Source: CAD feature listing. Evaluate the final solid. Frame: model axes, mm. A direction names the side the tool comes from. Round coordinates to 2 decimals unless told otherwise and drop trailing zeros. Write each loop counter-clockwise with the first axis right and the second up, starting at its lowest first coordinate (ties: lowest second). Pieces come first, ordered by that corner, then holes.
from build123d import *

# Parameters (mm, degrees)
SKETCH_1_R      = 1.65
EXTRUDE_1_DEPTH = 5
FILLET_2_R      = 4
FILLET_3_R      = 40
FILLET_4_R      = 10
EXTRUDE_2_DEPTH = 55


with BuildPart() as part:
    # 草图1 → 凸台-拉伸1 (new body)
    with BuildSketch(Plane.XY):
        with BuildLine():
            Line((-11.5, 79.5), (-11.5, 82))
            ThreePointArc((-11.5, 82), (6.103622298, 73.512939805), (10.426977744, 54.454442843))
            Line((10.426977744, 54.454442843), (13.41461423, 33.96926032))
            Line((13.41461423, 33.96926032), (11.539893904, 12.741041785))
            Line((11.539893904, 12.741041785), (4.278741136, 12.025251419))
            Line((4.278741136, 12.025251419), (-1.047111461, 14.664575003))
            Line((-1.047111461, 14.664575003), (3.709660575, 42.919402146))
            ThreePointArc((3.709660575, 42.919402146), (1.596827744, 41.204560595), (-0.707567867, 39.757320125))
            Line((-0.707567867, 39.757320125), (-1.906726993, 41.950951222))
            ThreePointArc((-1.906726993, 41.950951222), (7.877576933, 64.450708254), (-11.5, 79.5))
        make_face()
        with Locations((5.679475492, 16.683750627)):
            Circle(SKETCH_1_R, mode=Mode.SUBTRACT)
        with Locations((8.382327473, 29.399669437)):
            Circle(SKETCH_1_R, mode=Mode.SUBTRACT)
    extrude(amount=EXTRUDE_1_DEPTH)

    # 圆角2
    fillet_2_edges = [part.edges().sort_by_distance(p)[0] for p in [
        (10.426977744, 54.454442843, 2.5),
    ]]
    fillet(fillet_2_edges, radius=FILLET_2_R)

    # 圆角3
    fillet_3_edges = [part.edges().sort_by_distance(p)[0] for p in [
        (13.41461423, 33.96926032, 2.5),
    ]]
    fillet(fillet_3_edges, radius=FILLET_3_R)

    # 圆角4
    fillet_4_edges = [part.edges().sort_by_distance(p)[0] for p in [
        (4.278741136, 12.025251419, 2.5),
    ]]
    fillet(fillet_4_edges, radius=FILLET_4_R)

    # 草图2 → 凸台-拉伸2 (add)
    with BuildSketch(Plane(origin=(0, 0, 0), x_dir=(-1, 0, 0), z_dir=(0, 0, -1))):
        with BuildLine():
            Line((11.5, 82), (11.5, 79.5))
            ThreePointArc((11.5, 79.5), (-7.877576933, 64.450708254), (1.906726993, 41.950951222))
            Line((1.906726993, 41.950951222), (0.707567867, 39.757320125))
            ThreePointArc((0.707567867, 39.757320125), (-10.299774049, 65.069546786), (11.5, 82))
        make_face()
    extrude(amount=-EXTRUDE_2_DEPTH)


solid = part.part
1) Section query D-D on y = 74.5. Return the cut outline in (x, z).
Taken from the geometry:
outline: (1.73, 0) - (5.27, 0) - (5.27, 55) - (1.73, 55) - close
2) Section query C-C on y = 48.5. Return the cut outline in (x, z).
Taken from the geometry:
outline: (5.2, 0) - (11.3, 0) - (11.3, 5) - (8.13, 5) - (8.13, 55) - (5.2, 55) - close
3) Contact query for flat-ended pins moving along their axis: P1, Ø3, axis at y = 50, z = 7, coming from the -X side; P2, Ø1, axis at x = 4, y = 19.5, coming from the +Z side; P3, Ø1, axis at x = 4.5, z = 21.5, coming from the -Y side. Output: stop coordinate, or through.
Taken from the geometry:
P1: stops at x = 5.2
P2: stops at z = 5
P3: stops at y = 43.19
4) Pull-direction query (Y, two-part tool) for faces 1 (the face through (8.02, 27.79, 2.46)), 2 (the face through (9.367, 12.527, 2.465)), 3 (the face through (5, 37, 0)); classes: released by +Y, released by -Y, zero draft, split by the parting line, or undercut.
Taken from the geometry:
face 1: undercut
face 2: released by -Y
face 3: zero draft
5) Section query B-B on z = 42. Return the cut outline in (x, y).
Taken from the geometry:
outline: (-11.5, 79.5) arc R20 cw to (-1.91, 41.95) - (-0.71, 39.76) arc R22.5 ccw to (-11.5, 82) - close
6) Reachability of faces 4 (the face through (11.62, 46.28, 2.46)), 5 (the face through (-11.5, 81, 27)), 6 (the face through (6, 29, 5)) from +Z, -Z, +X, -X, +Y, -Y: full face, straight path, thin tool, end or side. Return the list, or none.
Taken from the geometry:
face 4: +Z, -Z, +X
face 5: +Z, -Z, -X, +Y, -Y
face 6: +Z, +X, -Y
7) Material intervals for line 1 (Z direction, x = 6.25, y = 23); line 2 (X direction, y = 60, z = 44); line 3 (Y direction, x = -0.5, z = 35.5), sorted ascending.
Taken from the geometry:
line 1: z = 0 to 5
line 2: x = 8.49 to 10.99
line 3: y = 39.87 to 42.8, 76.2 to 79.13
8) Section query A-A on x = 5.75. Return the cut outline in (y, z).
Taken from the geometry:
outline: (12.27, 0) - (15.04, 0) - (15.04, 5) - (12.27, 5) - close; (18.33, 0) - (49.38, 0) - (49.38, 55) - (45.05, 55) - (45.05, 5) - (18.33, 5) - close; (69.62, 0) - (73.95, 0) - (73.95, 55) - (69.62, 55) - close
